Here's how the part is built. I have some questions about the finished solid (model axes, mm). A direction names the side the tool comes from. Give positions to 0.01 mm unless a question says otherwise; leave off trailing zeros. Write each loop counter-clockwise with the first axis right and the second up, starting at its lowest first coordinate (ties: lowest second). Pieces come first, ordered by that corner, then holes. Notation, with made-up numbers: (-40, -40) - (7, -40) arc R12 ccw to (7, -21) - close; hole circle Ø9 at (14, 44.5). An arc over 180 degrees is marked (long way). Use a Markdown table: item, result.
Autodesk Inventor part; units mm, degrees
ref_plane "YZ Plane" through (0, 0, 0) normal (1, 0, 0) x (0, 1, 0)
ref_plane "XZ Plane" through (0, 0, 0) normal (0, 1, 0) x (-1, 0, 0)
ref_plane "XY Plane" through (0, 0, 0) normal (0, 0, 1) x (1, 0, 0)
sketch "Sketch1" plane through (0, 0, 0) normal (0, 0, 1) x (1, 0, 0)
  circle A0 centre (0, 0) radius 171.45
  dimension "d0" = 342.9
extrude "Extrusion1" add sketch "Sketch1" along normal blind 6.35
sketch "Sketch2" plane through (0, 0, 6.35) normal (0, 0, 1) x (1, 0, 0)
  circle A0 centre (0, 0) radius 171.45
  line L0 (197.6462, 0) -> (-281.2915, 0)
  line L1 (0, -189.9673) -> (0, 254.2486)
  line L2 (0, 0) -> (-224.0806, 224.0806)
  line L3 (-117.1025, 117.1025) -> (25.0798, 259.2849)
  line L4 (25.0798, 259.2849) -> (-193.4238, 635.0058)
  line L5 (-193.4238, 635.0058) -> (-427.1769, 145.6409)
  line L6 (-427.1769, 145.6409) -> (-369.1953, -134.9902)
  line L7 (-369.1953, -134.9902) -> (-88.5642, 145.6409)
  dimension "d3" = 45
  dimension "d4" = 165.608
extrude "Extrusion2" cut sketch "Sketch2" against normal blind 40 contours L3 L2 A0 | A0 L7 L6 L5 L4 L3 | L7 A0 L2
pattern_circular "Circular Pattern1" count 4 over 360 about axis through (0, 0, -10) along (0, 0, 1) of "Extrusion2"
sketch "Sketch3" plane through (0, 0, 6.35) normal (0, 0, 1) x (1, 0, 0)
  arc A0 (148.48, -85.7251) -> (148.48, 85.7251) centre (0, 0) ccw
  circle A1 centre (0, 0) radius 3.0226
  dimension "d10" = 6.0452
extrude "Extrusion3" cut sketch "Sketch3" against normal blind 40
sketch "Sketch4" plane through (0, 0, 6.35) normal (0, 0, 1) x (1, 0, 0)
  circle A0 centre (0, 0) radius 3.0226
  circle A1 centre (-163.83, 70.358) radius 38.1
  circle A2 centre (-70.358, 163.83) radius 38.1
  dimension "d13" = 76.2
  dimension "d14" = 76.2
  dimension "d15" = 70.358
  dimension "d16" = 70.358
  dimension "d17" = 163.83
  dimension "d18" = 163.83
extrude "Extrusion4" cut sketch "Sketch4" against normal blind 40 contours A1 | A2
fillet "Fillet1" radius 6.35 1 edges at (-136.8978, 97.3073, 3.175)
fillet "Fillet2" radius 6.35 1 edges at (-168.3366, 32.5255, 3.175)
fillet "Fillet3" radius 6.35 1 edges at (-97.3073, 136.8978, 3.175)
fillet "Fillet4" radius 6.35 1 edges at (-32.5255, 168.3366, 3.175)
sketch "Sketch5" plane through (0, 0, 6.35) normal (0, 0, 1) x (1, 0, 0)
  arc A0 (-169.3248, 26.9115) -> (-148.48, -85.7251) centre (0, 0) ccw
  circle A1 centre (0, 101.6) radius 4.9022
  dimension "d25" = 9.8044
  dimension "d26" = 101.6
extrude "Extrusion5" cut sketch "Sketch5" against normal blind 40
pattern_circular "Circular Pattern2" count 4 over 360 about axis through (0, 0, -10) along (0, 0, 1) of "Extrusion5"
sketch "Sketch6" plane through (0, 0, 6.35) normal (0, 0, 1) x (1, 0, 0)
  arc A0 (-169.3248, 26.9115) -> (-148.48, -85.7251) centre (0, 0) ccw
  circle A1 centre (0, 0) radius 3.0226
  circle A2 centre (-99.4768, 123.952) radius 2.159
  line L0 (0, 0) -> (-213.9537, 213.9537)
  circle A3 centre (0, 0) radius 3.0226
  line L1 (0, 0) -> (0, 193.7824)
  line L2 (-75.5206, 147.9082) -> (-146.0285, 77.4003)
  circle A4 centre (-111.7144, 111.7144) radius 2.159
  circle A5 centre (-123.952, 99.4768) radius 2.159
  line L3 (0, 0) -> (-99.4768, 123.952)
  line L4 (0, 0) -> (-123.952, 99.4768)
  dimension "d32" = 4.318
  dimension "d33" = 45
  dimension "d34" = 157.988
  dimension "d35" = 0
  dimension "d36" = 4.318
  dimension "d37" = 4.318
  dimension "d49" = 123.952
extrude "Extrusion6" cut sketch "Sketch6" against normal blind 40 contours L4 L2 A5 | A5 L2 L4 | L3 L2 A2 | A2 L2 L3 | A4 L2 L0 | L0 L2 A4 | A5 L2 | A2 L2 | L2 A4 L0 | L0 A4 L2
sketch "Sketch7" plane through (0, 0, 6.35) normal (0, 0, 1) x (1, 0, 0)
  circle A0 centre (-111.7144, 111.7144) radius 2.159
  circle A1 centre (-99.4768, 123.952) radius 2.159
  circle A2 centre (-123.952, 99.4768) radius 2.159
  circle A3 centre (-99.4768, 123.952) radius 4.2164
  circle A4 centre (-111.7144, 111.7144) radius 4.2164
  circle A5 centre (-123.952, 99.4768) radius 4.2164
  dimension "d41" = 8.4328
  dimension "d42" = 8.4328
  dimension "d43" = 8.4328
extrude "Extrusion7" cut sketch "Sketch7" against normal blind 2.54
pattern_circular "Circular Pattern3" count 4 over 360 about axis through (0, 0, -10) along (0, 0, 1) of "Extrusion6", "Extrusion7"
sketch "Sketch13" plane through (0, 0, 6.35) normal (0, 0, 1) x (1, 0, 0)
  circle A0 centre (101.6, 0) radius 4.9022
  circle A1 centre (0, 0) radius 3.0226
  line L0 (220.5677, -64) -> (53, -64)
  line L1 (53, -64) -> (53, 64)
  line L2 (53, 64) -> (220.5677, 64)
  line L3 (220.5677, 64) -> (220.5677, -64)
  line L4 (0, 0) -> (36.6997, 0) construction
  line L5 (0, 0) -> (0, -29.3606) construction
  line L6 (53, 64) -> (43, 14.6803)
  line L7 (43, 14.6803) -> (37, 0)
  line L8 (53, -64) -> (43, -14.6803)
  line L9 (43, -14.6803) -> (37, 0)
  arc A2 (148.48, -85.7251) -> (148.48, 85.7251) centre (0, 0) ccw
  dimension "d81" = 128
  dimension "d87" = 10
  dimension "d88" = 16
  dimension "d89" = 37
extrude "Extrusion11" cut sketch "Sketch13" against normal through all contours L0 A2 L2 L3 | L0 L1 L2 A2 | L8 L9 L7 L6 L1
fillet "Fillet7" radius 40 2 edges at (43, 14.6803, 3.175) (43, -14.6803, 3.175)
fillet "Fillet8" radius 3 2 edges at (53, -64, 3.175) (53, 64, 3.175)
sketch "Sketch14" plane through (0, 0, 6.35) normal (0, 0, 1) x (1, 0, 0)
  arc A0 (159.0569, 64) -> (148.48, 85.7251) centre (0, 0) ccw
  circle A1 centre (0, 0) radius 3.0226
  line L0 (41, -102) -> (-41, -102)
  line L1 (-41, -102) -> (-41, -54)
  line L2 (-41, -54) -> (41, -54)
  line L3 (41, -54) -> (41, -102)
  line L4 (0, 0) -> (0, -193.6891)
  dimension "d90" = 82
  dimension "d91" = 48
  dimension "d92" = 54
extrude "Extrusion12" cut sketch "Sketch14" against normal blind 20 contours L2 L3 L0 L4 | L4 L0 L1 L2
fillet "Fillet9" radius 3 1 edges at (37, 0, 3.175)
fillet "Fillet10" radius 3 4 edges at (-41, -54, 3.175) (41, -54, 3.175) (41, -102, 3.175) (-41, -102, 3.175)
fillet "Fillet11" radius 2 2 edges at (4.8859, -102, 3.175) (-4.8859, -102, 3.175)
fillet "Fillet12" radius 6.5 2 edges at (159.0569, -64, 3.175) (159.0569, 64, 3.175)
properties part number "Deck"
Item 1: I need wall thicknesses on line 1 along X through (y, z) = (-0.5, 3.5); line 2 along X through (y, z) = (-112.5, 6.25) (3 decimals); line 3 along Y through (x, z) = (-114, 4.5) (3 decimals). Which ranges of each line are inside material? Lowest first, please. Write a range as [from, to].
Values:
| item | result |
|---|---|
| line 1 | x = [-171.45, -106.48], [-96.72, -2.98], [2.98, 37.28] |
| line 2 | x = [-121.705, -115.857], [-107.572, 107.572], [115.857, 121.705] |
| line 3 | y = [-120.205, -115.258], [-108.171, 108.171], [115.258, 120.205] |
Item 2: If we section it at C-C, the plane y = -43.5: Write out the boundary of the cut face in (x, z), plus the area to 3 significant figures.
Values:
| item | result |
|---|---|
| outline | (-165.84, 0) - (48.84, 0) - (48.84, 6.35) - (-165.84, 6.35) - close |
| area | 1,360 mm2 |
Item 3: If we section it at D-D, the plane x = -46: Write out the boundary of the cut face in (y, z), plus the area to 3 significant figures.
Values:
| item | result |
|---|---|
| outline | (-165.16, 0) - (134.53, 0) - (134.53, 6.35) - (-165.16, 6.35) - close |
| area | 1,900 mm2 |
Item 4: If we section it at B-B, the plane z = 5: Count the separate pieces of the cut face and the enclosed holes in it, plus the area to 3 significant figures.
Values:
| item | result |
|---|---|
| separate pieces | 1 |
| enclosed holes | 16 |
| area | 67,300 mm2 |
Item 5: If we section it at A-A, the plane x = 90: Write out the boundary of the cut face in (y, z), plus the area to 3 significant figures.
Values:
| item | result |
|---|---|
| outline | (-144.21, 0) - (-64, 0) - (-64, 6.35) - (-144.21, 6.35) - close; (64, 0) - (144.21, 0) - (144.21, 6.35) - (64, 6.35) - close |
| area | 1,020 mm2 |
Item 6: Thinking about a two-plate mould opening in X: for faces 3 (the cylindrical face through (1.257, -171.445, 3.131)), 4 (the cylindrical face through (-168.437, -32.003, 3.131)), 5 (the cylindrical face through (-107.974, -109.769, 5.098)), which applies, +X half, -X half, draft (parallel to the pull), parting line (faces both ways), or undercut?
Values:
| item | result |
|---|---|
| face 3 | parting line |
| face 4 | -X half |
| face 5 | undercut |
Item 7: For faces 1 (the cylindrical face through (-54.13, 129.36, 3.22)), 2 (the cylindrical face through (-127.298, 96.911, 5.098)), which set-ups out of +Z, -Z, +X, -X, +Y, -Y let a thin tool reach every point of the face, with its end or its side?
Values:
| item | result |
|---|---|
| face 1 | +Z, -Z, +Y |
| face 2 | +Z |
Item 8: Will these pins go through, and if not, where does the flat tip stop? pin 1 Ø4 at (x, y) = (-112.5, 112) entering from +Z; pin 2 Ø2 at (x, z) = (78, 3) entering from -Y; pin 3 Ø1.5 at (y, z) = (125.5, 4) entering from -X (3 decimals).
Values:
| item | result |
|---|---|
| pin 1 | stops at z = 3.81 |
| pin 2 | stops at y = -153.19 |
| pin 3 | stops at x = -109.455 |
